```python
from build123d import *

# Parameters (mm, degrees)
BOARD_OUTLINE_DEPTH = 0.508
SKETCH2_R           = 0.0762
NPTH_DEPTH          = 1.508
SKETCH3_R           = 0.405
PTH_DEPTH           = 1.508


with BuildPart() as part:
    # Sketch1 → Board_Outline (new body)
    with BuildSketch(Plane.XY):
        Polygon((0, 0), (0, 20.955), (1.5875, 22.5425), (11.1125, 22.5425), (12.7, 20.955), (12.7, 0), align=None)
    extrude(amount=BOARD_OUTLINE_DEPTH)

    # Sketch2 → NPTH (cut, through all)
    with BuildSketch(Plane.XY):
        with Locations((10.287, 8.3312)):
            Circle(SKETCH2_R)
        with Locations((7.6708, 4.2418)):
            Circle(SKETCH2_R)
        with Locations((6.731, 19.812)):
            Circle(SKETCH2_R)
        with Locations((11.2014, 15.6464)):
            Circle(SKETCH2_R)
        with Locations((5.3086, 19.812)):
            Circle(SKETCH2_R)
        with Locations((2.5654, 16.3576)):
            Circle(SKETCH2_R)
        with Locations((4.699, 19.812)):
            Circle(SKETCH2_R)
        with Locations((3.0734, 17.0688)):
            Circle(SKETCH2_R)
        with Locations((4.0894, 19.812)):
            Circle(SKETCH2_R)
        with Locations((3.5814, 18.1864)):
            Circle(SKETCH2_R)
        with Locations((8.5598, 19.812)):
            Circle(SKETCH2_R)
        with Locations((8.6614, 16.9672)):
            Circle(SKETCH2_R)
        with Locations((7.9502, 19.812)):
            Circle(SKETCH2_R)
        with Locations((9.1694, 18.1864)):
            Circle(SKETCH2_R)
        with Locations((7.3406, 19.812)):
            Circle(SKETCH2_R)
        with Locations((10.0838, 16.4592)):
            Circle(SKETCH2_R)
        with Locations((6.0198, 19.812)):
            Circle(SKETCH2_R)
        with Locations((2.159, 15.8496)):
            Circle(SKETCH2_R)
        with Locations((4.699, 7.112)):
            Circle(SKETCH2_R)
        with Locations((3.175, 5.588)):
            Circle(SKETCH2_R)
        with Locations((4.3942, 3.4544)):
            Circle(SKETCH2_R)
        with Locations((2.9718, 4.8768)):
            Circle(SKETCH2_R)
        with Locations((5.5118, 7.112)):
            Circle(SKETCH2_R)
        with Locations((6.5278, 6.8072)):
            Circle(SKETCH2_R)
        with Locations((6.5278, 3.048)):
            Circle(SKETCH2_R)
        with Locations((9.6774, 2.6416)):
            Circle(SKETCH2_R)
        with Locations((7.5438, 7.0104)):
            Circle(SKETCH2_R)
        with Locations((5.1054, 6.1976)):
            Circle(SKETCH2_R)
        with Locations((9.779, 3.7592)):
            Circle(SKETCH2_R)
        with Locations((8.9662, 6.2992)):
            Circle(SKETCH2_R)
        with Locations((8.763, 7.112)):
            Circle(SKETCH2_R)
        with Locations((8.1534, 6.5024)):
            Circle(SKETCH2_R)
        with Locations((8.0518, 5.3848)):
            Circle(SKETCH2_R)
        with Locations((1.3462, 10.7696)):
            Circle(SKETCH2_R)
        with Locations((10.8712, 6.985)):
            Circle(SKETCH2_R)
    extrude(amount=NPTH_DEPTH, mode=Mode.SUBTRACT)

    # Sketch3 → PTH (cut, through all)
    with BuildSketch(Plane.XY):
        with Locations((2.22, 18.1)):
            Circle(SKETCH3_R)
        with Locations((10.48, 18.1)):
            Circle(SKETCH3_R)
        with Locations((1.91, 1.27)):
            Circle(SKETCH3_R)
    extrude(amount=PTH_DEPTH, mode=Mode.SUBTRACT)


solid = part.part
```
Geometry: final body of the model. Coordinates: model frame, mm. Coordinates: 2 decimals unless noted, no trailing zeros. Loops run counter-clockwise (first coordinate to the right, second up) from the corner with the lowest first, then second, coordinate; pieces in that order, holes last. Notation, with made-up numbers: (17, 83) -> (45, 83) arc R30 cw to (45, 119) -> close; hole circle Ø3 at (0.5, 76). An arc over 180 degrees is marked (long way). Use a Markdown table: item, result. Add a question column.
(1) Section query A-A, the plane y = 1.27. Return loops of the section in (x, z) (3 decimals), plus the area to 3 significant figures.
(2) Section query B-B, the plane z = 0.35. State how many separate pieces and enclosed holes the cut face has, plus the area to 3 significant figures.
(3) Line query: line 1 along X through (y, z) = (1.27, 0.3) (3 decimals); line 2 along Y through (x, z) = (10.48, 0.35) (1 decimal); line 3 along Y through (x, z) = (2, 0.1). Output: solid intervals per line, ascending.
(4) Mould query, pull axis Y, two halves, no side actions, for faces 1 (the cylindrical face through (10.18, 18.37, 0.25)), 2 (the flat face through (11.895, 21.76, 0.25)), 3 (the flat face through (6, 11, 0.508)). Classes: pulls with the +Y half, pulls with the -Y half, needs draft (parallel to the pull), parting line crosses it, or undercut.
Answer:
| question | item | result |
|---|---|---|
| 1 | outline | (0, 0) -> (1.505, 0) -> (1.505, 0.508) -> (0, 0.508) -> close; (2.315, 0) -> (12.7, 0) -> (12.7, 0.508) -> (2.315, 0.508) -> close |
| 1 | area | 6.04 mm^2 |
| 2 | separate pieces | 1 |
| 2 | enclosed holes | 38 |
| 2 | area | 282 mm^2 |
| 3 | line 1 | x = 0 to 1.505, 2.315 to 12.7 |
| 3 | line 2 | y = 0 to 17.7, 18.5 to 22.5 |
| 3 | line 3 | y = 0 to 0.88, 1.66 to 17.76, 18.44 to 22.54 |
| 4 | face 1 | undercut |
| 4 | face 2 | pulls with the +Y half |
| 4 | face 3 | needs draft |
